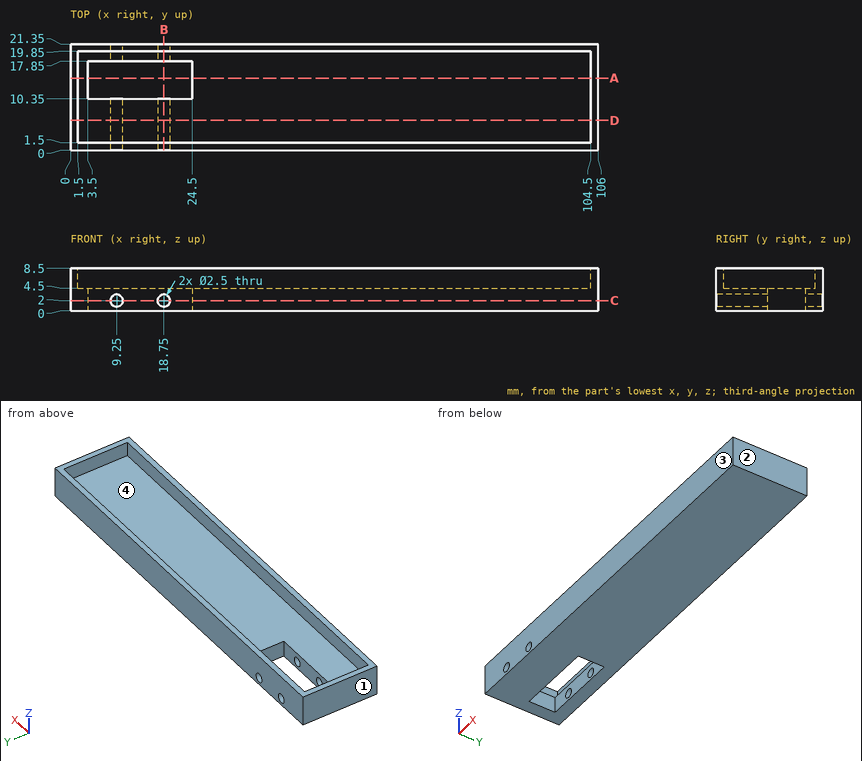
Check sheet for the drawn part. Datum: minimum x, y, z corner. Units: mm. Round coordinates to 2 decimals unless told otherwise and drop trailing zeros. Order: outer loops, then holes, each group sorted by start corner. A loop starts at its lowest first (then second) coordinate and runs counter-clockwise, first axis right, second up. Notation, with made-up numbers: (56, 88.25) -> (104, 88.25) arc R24 ccw to (104, 117.25) -> close; hole circle Ø5 at (-24, 27.5). An arc over 180 degrees is marked (long way). Return JSON: item names as keys, results as strings. Group by question number.
Q1. Gauge pin test, flat end, axial feed: pin 1 (3 mm diameter, centred on x = 88.5, y = 5, fed in from +Z). Record the tip position at first contact, or that the pin passes through.
Q2. Section check D-D, the plane y = 6. Record the boundary of the cut face in (x, z).
Q3. Section check B-B, the plane x = 18.75. Record the boundary of the cut face in (y, z).
Q4. Section check C-C, the plane z = 2. Record the boundary of the cut face in (x, y), plus the area to 3 significant figures.
Q5. Material ranges on probe 1 along X at (y, z) = (6, 2); probe 2 along Y at (x, z) = (77.5, 4.75); probe 3 along X at (y, z) = (13.5, 2.5), recorded low to high. Write a range as from..to.
Q6. Section check A-A, the plane y = 14.5. Record the boundary of the cut face in (x, z).
Q7. Release check for a two-part mould opening along X. For the marked faces 1, 2, 3 and 4 record: released by +X, released by -X, zero draft, split by the parting line, or undercut.
Numbers:
{
 "1": {"pin 1": "z = 4.5"},
 "2": {"outline": "(0, 0) -> (106, 0) -> (106, 8.5) -> (104.5, 8.5) -> (104.5, 4.5) -> (1.5, 4.5) -> (1.5, 8.5) -> (0, 8.5) -> close; hole circle Ø2.5 at (9.25, 2); hole circle Ø2.5 at (18.75, 2)"},
 "3": {"outline": "(0, 0) -> (10.35, 0) -> (10.35, 0.75) -> (0, 0.75) -> close; (0, 3.25) -> (10.35, 3.25) -> (10.35, 4.5) -> (1.5, 4.5) -> (1.5, 8.5) -> (0, 8.5) -> close; (17.85, 0) -> (21.35, 0) -> (21.35, 0.75) -> (17.85, 0.75) -> close; (17.85, 3.25) -> (21.35, 3.25) -> (21.35, 8.5) -> (19.85, 8.5) -> (19.85, 4.5) -> (17.85, 4.5) -> close"},
 "4": {"outline": "(0, 0) -> (8, 0) -> (8, 10.35) -> (3.5, 10.35) -> (3.5, 17.85) -> (8, 17.85) -> (8, 21.35) -> (0, 21.35) -> close; (10.5, 0) -> (17.5, 0) -> (17.5, 10.35) -> (10.5, 10.35) -> close; (10.5, 17.85) -> (17.5, 17.85) -> (17.5, 21.35) -> (10.5, 21.35) -> close; (20, 0) -> (106, 0) -> (106, 21.35) -> (20, 21.35) -> (20, 17.85) -> (24.5, 17.85) -> (24.5, 10.35) -> (20, 10.35) -> close", "area": "2,040 mm^2"},
 "5": {"probe 1": "0..8, 10.5..17.5, 20..106", "probe 2": "0..1.5, 19.85..21.35", "probe 3": "0..3.5, 24.5..106"},
 "6": {"outline": "(0, 0) -> (3.5, 0) -> (3.5, 4.5) -> (1.5, 4.5) -> (1.5, 8.5) -> (0, 8.5) -> close; (24.5, 0) -> (106, 0) -> (106, 8.5) -> (104.5, 8.5) -> (104.5, 4.5) -> (24.5, 4.5) -> close"},
 "7": {"face 1": "released by -X", "face 2": "released by +X", "face 3": "zero draft", "face 4": "undercut"}
}
